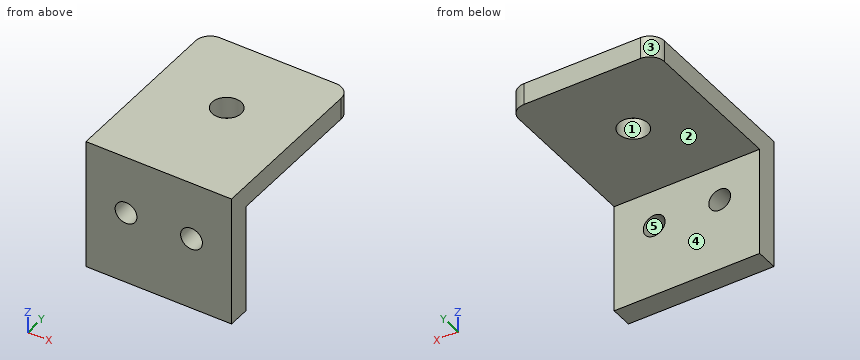
from build123d import *

# Parameters (mm, degrees)
EXTRUDE_1_DEPTH     = 20
SKETCH_2_R          = 1.5
CUT_EXTRUDE_1_DEPTH = 35.756294394
FILLET_1_R          = 2
SKETCH_3_R          = 2
CUT_EXTRUDE_2_DEPTH = 37.728735344


with BuildPart() as part:
    # 草图1 → 凸台-拉伸1 (new body)
    with BuildSketch(Plane(origin=(0, 0, 0), x_dir=(0, 0, -1), z_dir=(1, 0, 0))):
        Polygon((0, 0), (0, 25), (3, 25), (3, 3), (18, 3), (18, 0), align=None)
    extrude(amount=EXTRUDE_1_DEPTH)

    # 草图2 → 切除-拉伸1 (cut, through all)
    with BuildSketch(Plane(origin=(0, 3, 0), x_dir=(1, 0, 0), z_dir=(0, 1, 0))):
        with Locations(Location((5.5, 8, 0), (0, 0, 270))):
            Circle(SKETCH_2_R)
        with Locations(Location((14.5, 8, 0), (0, 0, 270))):
            Circle(SKETCH_2_R)
    extrude(amount=-CUT_EXTRUDE_1_DEPTH, mode=Mode.SUBTRACT)

    # 圆角1
    fillet_1_edges = [part.edges().sort_by_distance(p)[0] for p in [
        (20, 25, -1.5),
        (0, 25, -1.5),
    ]]
    fillet(fillet_1_edges, radius=FILLET_1_R)

    # 草图3 → 切除-拉伸2 (cut, through all)
    with BuildSketch(Plane.XY):
        with Locations((10, 14.25)):
            Circle(SKETCH_3_R)
    extrude(amount=-CUT_EXTRUDE_2_DEPTH, mode=Mode.SUBTRACT)


solid = part.part
Can you work these out from the model? Positions are in its coordinate system, mm. Face numbers are marked on the shaded views. A direction names the side the tool comes from. Coordinates: 2 decimals unless noted, no trailing zeros. Write each loop counter-clockwise with the first axis right and the second up, starting at its lowest first coordinate (ties: lowest second). Pieces come first, ordered by that corner, then holes.
Q1. Imagine slicing it at A-A, the plane x = 14.5. List the corners of the cut face in (y, z) for me.
Results found:
outline: (0, -18) - (3, -18) - (3, -9.5) - (0, -9.5) - close; (0, -6.5) - (3, -6.5) - (3, -3) - (25, -3) - (25, 0) - (0, 0) - close
Q2. For P1, Ø6, axis at x = 6.5, y = 14.5, coming from the -Z side; P2, Ø3, axis at x = 17.5, z = -13, coming from the +Y side, each with a flat end and sliding along its axis, tell me the tip position at first contact or that it passes through.
Results found:
P1: stops at z = -3
P2: stops at y = 3
Q3. Imagine slicing it at D-D, the plane z = -8.25. List the corners of the cut face in (x, y) for me, plus the area to 3 significant figures.
Results found:
outline: (0, 0) - (4.02, 0) - (4.02, 3) - (0, 3) - close; (6.98, 0) - (13.02, 0) - (13.02, 3) - (6.98, 3) - close; (15.98, 0) - (20, 0) - (20, 3) - (15.98, 3) - close
area: 42.3 mm2
Q4. Please list where these lines run through material, in increasing order: L1, parallel to X at y = 2.05, z = -8; L2, parallel to Y at x = 10, z = -1.1; L3, parallel to Y at x = 6, z = -5.5.
Results found:
L1: x = 0 to 4, 7 to 13, 16 to 20
L2: y = 0 to 12.25, 16.25 to 25
L3: y = 0 to 3
Q5. Which directions (+Z, -Z, +X, -X, +Y, -Y) give clear straight access to the entire face, cutting with the end or side of a thin tool? Please do the marked faces 4 and 5.
Results found:
face 4: -Z, +X, -X, +Y
face 5: +Y, -Y
Q6. Imagine slicing it at B-B, the plane y = 14.25. List the corners of the cut face in (x, z) for me.
Results found:
outline: (0, -3) - (8, -3) - (8, 0) - (0, 0) - close; (12, -3) - (20, -3) - (20, 0) - (12, 0) - close
Q7. Imagine slicing it at C-C, the plane z = -1.5. List the corners of the cut face in (x, y) for me.
Results found:
outline: (0, 0) - (20, 0) - (20, 23) arc R2 ccw to (18, 25) - (2, 25) arc R2 ccw to (0, 23) - close; hole circle Ø4 at (10, 14.25)
Q8. If we mould it in two halves opening along X, with no side actions, what happens to the marked faces 1, 2 and 3? For each: +X half, -X half, draft (parallel to the pull), parting line (faces both ways), or undercut.
Results found:
face 1: undercut
face 2: draft
face 3: -X half
